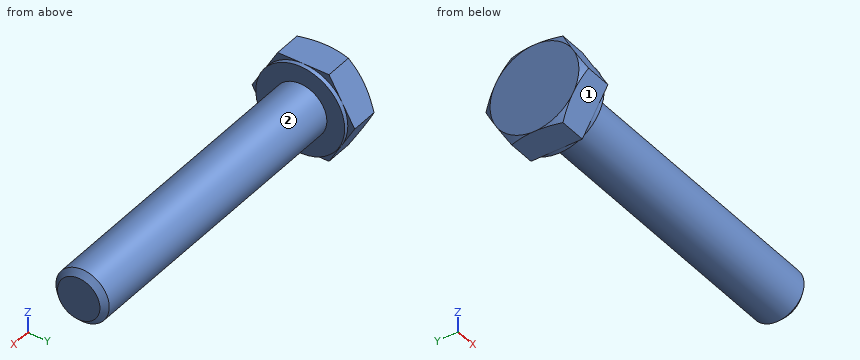
Autodesk Inventor part; units mm, degrees
ref_plane "Work Plane1" through (1.525, 0, 0) normal (0, 0, 1) x (1, 0, 0)
ref_plane "YZ Plane" through (0, 0, 0) normal (1, 0, 0) x (0, 1, 0)
ref_plane "XZ Plane" through (0, 0, 0) normal (0, 1, 0) x (-1, 0, 0)
sketch "Sketch1" plane through (0, 0, 0) normal (0, 0, 1) x (1, 0, 0)
  line L0 (0, 5) -> (0, 3)
  line L1 (3, 3) -> (35, 3)
  line L2 (35, 3) -> (35, 0)
  line L3 (35, 0) -> (-0.5001, 0)
  line L4 (-7.6001, 0) -> (42.1, 0)
  line L5 (-0.5001, 0) -> (-0.5001, 5)
  line L6 (-0.5001, 5) -> (0, 5)
  line L7 (3, 3) -> (2.3865, 3)
  line L8 (2.3865, 3) -> (0, 3)
  line L9 (0, -1) -> (0, 6)
  dimension "d0" = 35
  dimension "d1" = 32
  dimension "d2" = 6
  dimension "d9" = 0.5001
  dimension "d10" = 10
  dimension "d13" = 0.6136
  dimension "d14" = 6
revolve "Body" add sketch "Sketch1" angle 360 about axis through (35, 0, 0) along (-1, 0, 0)
sketch "Sketch2" plane through (-0.5001, 0, 0) normal (-1, 0, 0) x (0, 0, 1)
  line L0 (0, 5.7735) -> (5, 2.8868)
  line L1 (5, 2.8868) -> (5, -2.8868)
  line L2 (5, -2.8868) -> (0, -5.7735)
  line L3 (0, -5.7735) -> (-5, -2.8868)
  line L4 (-5, -2.8868) -> (-5, 2.8868)
  line L5 (-5, 2.8868) -> (0, 5.7735)
  point P0 (0, 0)
  point P1 (0, 0)
  dimension "d11" = 10
extrude "Head" add sketch "Sketch2" along normal blind 3.5
sketch "Sketch4" plane through (0, 0, 0) normal (0, 0, 1) x (1, 0, 0)
  line L0 (-4.0001, 5) -> (-4.0001, 5.7735)
  line L1 (-4.0001, 5.7735) -> (-3.5535, 5.7735)
  line L2 (-3.5535, 5.7735) -> (-4.0001, 5)
  line L3 (-4.7001, 0) -> (0.1999, 0)
  line L4 (-0.5001, 5.7735) -> (-4.0001, 5.7735)
  line L5 (-4.0001, 2.8868) -> (-4.0001, 5.7735)
  dimension "d5" = 30
  dimension "d19" = 10
revolve "Chamfer1" cut sketch "Sketch4" angle 360 about axis through (-10, 0, 0) along (1, 0, 0)
thread "Thread"
chamfer "Chamfer2" distance 0.6135 distance2 0.6136 1 edges at (35, -3, 0) measured on face at (35, 0.7485, -0.6631)
ref_plane "Work Plane1" through (1.525, 0, 0) normal (0, 0, 1) x (1, 0, 0)
equation "\"d0\" = NLG"
equation "\"d1\" = GEL"
equation "\"d2\" = GD"
equation "\"d10\" = SD2"
equation "\"d14\" = BDM"
equation "\"d11\" = SW"
equation "\"d3\" = KOH - SD"
equation "\"d5\" = ANG1"
equation "\"d19\" = SW0"
equation "\"d15\" = GEL"
equation "\"d6\" = -0.5 * SPD + 0.5 * GD"
equation "\"NLG\" = 35"
equation "\"GD\" = NND"
equation "\"BDM\" = NND"
equation "\"KOH\" = 4"
equation "\"GEL\" = 32"
equation "\"SW\" = 10"
equation "\"SW0\" = SW"
equation "\"SPD\" = NND - 1.2269 * PTC"
equation "\"SD2\" = SW"
equation "\"SD\" = 0.5"
equation "\"ANG1\" = 30deg"
equation "\"GAL\" = 0.61345 * PTC"
equation "\"GUL\" = 0.61345 * PTC"
equation "\"RR\" = 0.25"
equation "\"WFT\" = SD"
equation "\"GD1\" = THREADDIA - 1.2269 * PTC"
equation "\"THREADDIA\" = 6"
equation "\"TOA\" = 30deg"
equation "\"FAWI\" = 45deg"
equation "\"PTC\" = 1"
equation "\"NND\" = 6"
equation "\"E0\" = 1.155 * SW"
properties part number "AS 1110 - M6 x 35" material "Steel, Mild"
Input: part model. Units: mm. Frame: model coordinates. Face numbers are marked on the shaded views. A direction names the side the tool comes from. Coordinates: 2 decimals unless noted, no trailing zeros. Write each loop counter-clockwise with the first axis right and the second up, starting at its lowest first coordinate (ties: lowest second). Pieces come first, ordered by that corner, then holes. Notation, with made-up numbers: (16, 48) - (72, 48) arc R12 cw to (72, 64) - close; hole circle Ø11 at (88.5, 61). An arc over 180 degrees is marked (long way). Put each result on its own line as item: value. Start each with the question number.
1) Reachability of the marked faces 1 and 2 from +Z, -Z, +X, -X, +Y, -Y: full face, straight path, thin tool, end or side. Return the list, or none.
2) Contact query for flat-ended pins moving along their axis: pin 1 (0.8 mm diameter, centred on y = 2, z = -3.5, fed in from +X); pin 2 (1.5 mm diameter, centred on x = 21.5, z = 0.5, fed in from -Y); pin 3 (2 mm diameter, centred on x = 27, z = -2, fed in from +Y). Output: stop coordinate, or through.
3) Ray query, L1, parallel to X at y = 2.5, z = -3.5; L2, parallel to X at y = 5.25, z = 0.5; L3, parallel to Y at x = 12, z = 0. Return the intervals inside material, ascending.
4) Cut plane A-A (x = 23). Return the cut outline in (y, z), plus the area to 3 significant figures.
Resolved:
1. face 1: -Z, +X, -X, -Y
1. face 2: +X
2. pin 1: stops at x = 0
2. pin 2: stops at y = -3
2. pin 3: stops at y = 2.83
3. L1: x = -4 to 0
3. L2: x = -3.84 to -0.5
3. L3: y = -3 to 3
4. outline: circle Ø6 at (0, 0)
4. area: 28.3 mm2
